```python
from build123d import *

# Parameters (mm, degrees)
BOX001_W                    = 3.5
BOX001_H                    = 11
BOX001_DEPTH                = 1.77
CYLINDER002_R               = 0.7
CYLINDER002_DEPTH           = 10
CYLINDER002_PLACEMENT_ANGLE = 92
CYLINDER007_R               = 0.7
CYLINDER007_DEPTH           = 10
CYLINDER007_ROLL_ANGLE      = 90
CYLINDER_R                  = 14
CYLINDER_DEPTH              = 13
THICKNESS_T                 = 1.77
CYLINDER003_R               = 1.5
CYLINDER003_DEPTH           = 10
CYLINDER004_R               = 1.5
CYLINDER004_DEPTH           = 10
CYLINDER005_R               = 1.5
CYLINDER005_DEPTH           = 10
CYLINDER006_R               = 1.5
CYLINDER006_DEPTH           = 10
CYLINDER001_R               = 14
CYLINDER001_DEPTH           = 10
BOX_W                       = 35.9
BOX_H                       = 35.9
BOX_DEPTH                   = 1.77


with BuildPart() as cube001:
    # Box001 → Box001 (new body)
    with BuildSketch(Plane(origin=(14.45, -5.5, 0), x_dir=(1, 0, 0), z_dir=(0, 0, 1))):
        with Locations((1.75, 5.5)):
            Rectangle(BOX001_W, BOX001_H)
    extrude(amount=BOX001_DEPTH)


with BuildPart() as cylinder002:
    # Cylinder002 → Cylinder002 (new body)
    with BuildSketch(Plane.XY):
        Circle(CYLINDER002_R)
    extrude(amount=CYLINDER002_DEPTH)


with BuildPart() as cylinder002_1:
    # Cylinder002 placement: moved
    add(cylinder002.part.moved(Location((12, 0, 10.7))).rotate(Axis((12, 0, 10.7), (0, 1, 0)), CYLINDER002_PLACEMENT_ANGLE))


with BuildPart() as cylinder007:
    # Cylinder007 → Cylinder007 (new body)
    with BuildSketch(Plane.XY):
        Circle(CYLINDER007_R)
    extrude(amount=CYLINDER007_DEPTH)


with BuildPart() as cylinder007_1:
    # Cylinder007 roll: moved
    add(cylinder007.part.rotate(Axis((0, 0, 0), (1, 0, 0)), CYLINDER007_ROLL_ANGLE))


with BuildPart() as cylinder007_2:
    # Cylinder007 placement: moved
    add(cylinder007_1.part.moved(Location((0, 21, 10.7))))


with BuildPart() as lens_conduit:
    # Cylinder → Cylinder (new body)
    with BuildSketch(Plane.XY):
        Circle(CYLINDER_R)
    extrude(amount=CYLINDER_DEPTH)

    # Thickness
    thickness_openings = [lens_conduit.faces().sort_by_distance(p)[0] for p in [
        (0, 0, 13),
        (0, 0, 0),
    ]]
    offset(amount=THICKNESS_T, openings=thickness_openings)

    # Cut005: cut Cylinder007
    add(cylinder007_2.part, mode=Mode.SUBTRACT)

    # Cut006: cut Cylinder002
    add(cylinder002_1.part, mode=Mode.SUBTRACT)

    # Cut008: cut Cube001
    add(cube001.part, mode=Mode.SUBTRACT)


with BuildPart() as cylinder003:
    # Cylinder003 → Cylinder003 (new body)
    with BuildSketch(Plane(origin=(13.5, 13.5, -2), x_dir=(1, 0, 0), z_dir=(0, 0, 1))):
        Circle(CYLINDER003_R)
    extrude(amount=CYLINDER003_DEPTH)


with BuildPart() as cylinder004:
    # Cylinder004 → Cylinder004 (new body)
    with BuildSketch(Plane(origin=(13.5, -13.5, -2), x_dir=(1, 0, 0), z_dir=(0, 0, 1))):
        Circle(CYLINDER004_R)
    extrude(amount=CYLINDER004_DEPTH)


with BuildPart() as cylinder005:
    # Cylinder005 → Cylinder005 (new body)
    with BuildSketch(Plane(origin=(-13.5, 13.5, -2), x_dir=(1, 0, 0), z_dir=(0, 0, 1))):
        Circle(CYLINDER005_R)
    extrude(amount=CYLINDER005_DEPTH)


with BuildPart() as cylinder006:
    # Cylinder006 → Cylinder006 (new body)
    with BuildSketch(Plane(origin=(-13.5, -13.5, -2), x_dir=(1, 0, 0), z_dir=(0, 0, 1))):
        Circle(CYLINDER006_R)
    extrude(amount=CYLINDER006_DEPTH)


with BuildPart() as cylinder001:
    # Cylinder001 → Cylinder001 (new body)
    with BuildSketch(Plane.XY.offset(-3)):
        Circle(CYLINDER001_R)
    extrude(amount=CYLINDER001_DEPTH)


with BuildPart() as fusion:
    # Box → Box (new body)
    with BuildSketch(Plane(origin=(-17.95, -17.95, 0), x_dir=(1, 0, 0), z_dir=(0, 0, 1))):
        with Locations((17.95, 17.95)):
            Rectangle(BOX_W, BOX_H)
    extrude(amount=BOX_DEPTH)

    # Cut: cut Cylinder001
    add(cylinder001.part, mode=Mode.SUBTRACT)

    # Cut001: cut Cylinder006
    add(cylinder006.part, mode=Mode.SUBTRACT)

    # Cut002: cut Cylinder005
    add(cylinder005.part, mode=Mode.SUBTRACT)

    # Cut003: cut Cylinder004
    add(cylinder004.part, mode=Mode.SUBTRACT)

    # Cut004: cut Cylinder003
    add(cylinder003.part, mode=Mode.SUBTRACT)

    # Cut007: cut Cube001
    add(cube001.part, mode=Mode.SUBTRACT)

    # Fusion: union lens_conduit
    add(lens_conduit.part)


solid = fusion.part
```
The listing builds one solid part. Answer for the finished solid, in the listing's coordinates (mm). A direction names the side the tool comes from. Round coordinates to 2 decimals unless told otherwise and drop trailing zeros. Loops run counter-clockwise (first coordinate to the right, second up) from the corner with the lowest first, then second, coordinate; pieces in that order, holes last.
1) Given P1, Ø3, axis at x = -2.5, z = 10, coming from the -Y side; P2, Ø0.9, axis at y = -1, z = 0.5, coming from the +X side; P3, Ø1.6, axis at x = 0, z = 10.7, coming from the -Y side, each flat-ended and moving along its own axis, determine where each tip first touches the part or whether it passes through.
Outcome:
P1: stops at y = -15.74
P2: stops at x = 14.45
P3: stops at y = -15.77
2) For a pull along Z with two mould halves and no side action, classify faces 1 (the face through (17.95, -12, 1)), 2 (the face through (-0.091, 14.889, 11.394)), 3 (the face through (-1.2, 14.1, 13)) as released by +Z, released by -Z, zero draft, split by the parting line, or undercut.
Outcome:
face 1: zero draft
face 2: undercut
face 3: released by +Z
3) For faces 4 (the face through (15, 0, 1.77)), 5 (the face through (14.9, 0, 11.3)), 6 (the face through (0, -17.95, 1)), 7 (the face through (-16, 0, 1.77)), determine the directions among +Z, -Z, +X, -X, +Y, -Y from which every point of the face is accessible in a straight line to the end or side of a thin tool.
Outcome:
face 4: -Z, +X
face 5: none
face 6: +Z, -Z, +X, -X, -Y
face 7: +Z
4) A cutting plane is placed at C-C on y = 13.5. Determine the outline of the cut face in (x, z), plus the area to 3 significant figures.
Outcome:
outline: (-17.95, 0) - (-15, 0) - (-15, 1.77) - (-17.95, 1.77) - close; (-12, 0) - (-3.71, 0) - (-3.71, 13) - (-8.15, 13) - (-8.15, 1.77) - (-12, 1.77) - close; (3.71, 0) - (12, 0) - (12, 1.77) - (8.15, 1.77) - (8.15, 13) - (3.71, 13) - close; (15, 0) - (17.95, 0) - (17.95, 1.77) - (15, 1.77) - close
area: 140 mm2
5) Consider line 1 (Z direction, x = -16, y = 1.5); line 2 (X direction, y = 5, z = 3.75); line 3 (X direction, y = -3, z = 8.5). Determine where each line is inside the solid, lowest interval first.
Outcome:
line 1: z = 0 to 1.77
line 2: x = -14.96 to -13.08, 13.08 to 14.96
line 3: x = -15.48 to -13.67, 13.67 to 15.48
6) A cutting plane is placed at B-B on x = -8. Determine the outline of the cut face in (y, z), plus the area to 3 significant figures.
Outcome:
outline: (-17.95, 0) - (-11.49, 0) - (-11.49, 13) - (-13.59, 13) - (-13.59, 1.77) - (-17.95, 1.77) - close; (11.49, 0) - (17.95, 0) - (17.95, 1.77) - (13.59, 1.77) - (13.59, 13) - (11.49, 13) - close
area: 70.1 mm2
7) A cutting plane is placed at A-A on y = -7. Determine the outline of the cut face in (x, z), plus the area to 3 significant figures.
Outcome:
outline: (-17.95, 0) - (-12.12, 0) - (-12.12, 13) - (-14.13, 13) - (-14.13, 1.77) - (-17.95, 1.77) - close; (12.12, 0) - (17.95, 0) - (17.95, 1.77) - (14.13, 1.77) - (14.13, 13) - (12.12, 13) - close
area: 65.7 mm2
